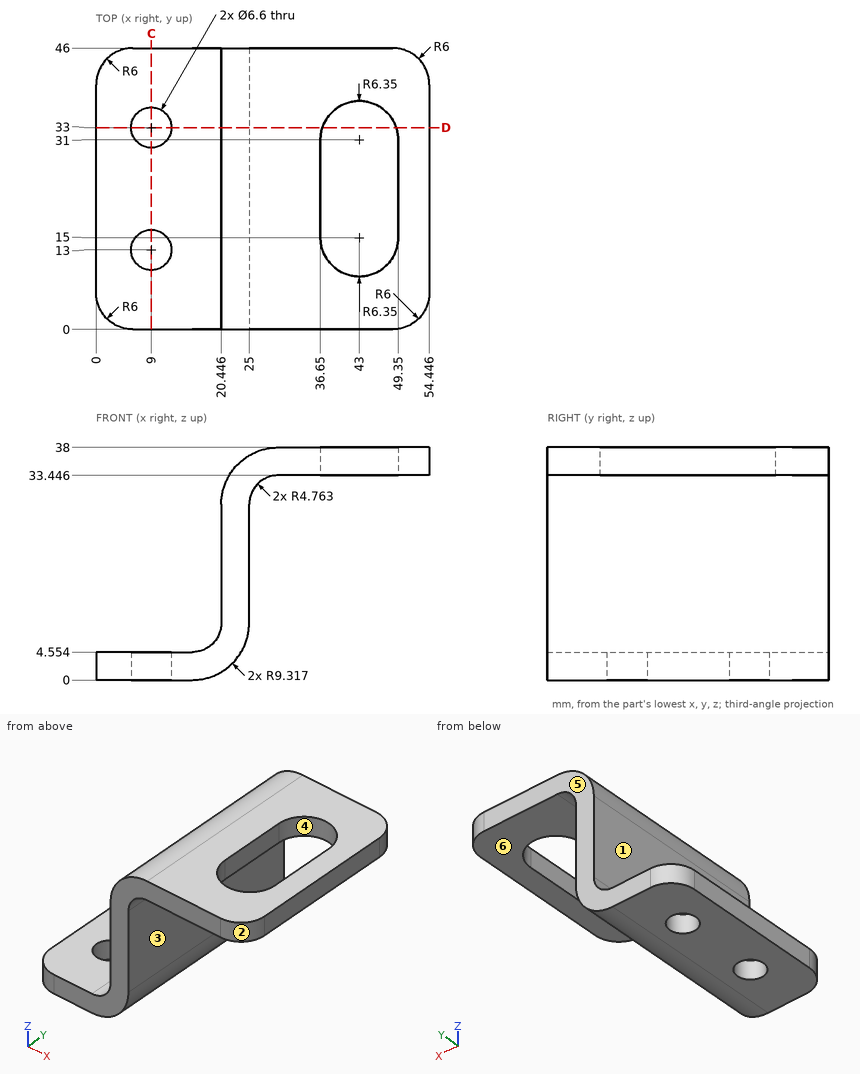
Input: dimensioned drawing with shaded views. Units: mm. Origin: part minimum x, y, z. A direction names the side the tool comes from. Give positions to 0.01 mm unless a question says otherwise; leave off trailing zeros. Write each loop counter-clockwise with the first axis right and the second up, starting at its lowest first coordinate (ties: lowest second). Pieces come first, ordered by that corner, then holes.
1. Reachability of the marked faces 1, 2 and 3 from +Z, -Z, +X, -X, +Y, -Y: full face, straight path, thin tool, end or side. Return the list, or none.
2. Section query C-C, the plane x = 9. Return loops of the section in (y, z) (1 decimal).
3. Line query: probe 1 along Y at (x, z) = (9, 2.4); probe 2 along X at (y, z) = (20, 11) (1 decimal); probe 3 along Z at (x, y) = (48, 35.5) (1 decimal). Output: solid intervals per line, ascending.
4. Section query D-D, the plane y = 33. Return loops of the section in (x, z) (1 decimal).
5. Draft query along Y for the marked faces 4, 5 and 6. Return one class per face: released by +Y, released by -Y, zero draft, split by the parting line, or undercut.
6. Pin query (flat end, axial travel): P1, Ø1.5, axis at x = 24.5, y = 23.5, coming from the +Z side (1 decimal); P2, Ø3, axis at y = 13.5, z = 31, coming from the -X side; P3, Ø3.5, axis at y = 21, z = 35, coming from the -X side. Return the tip coordinate at first contact, or that it passes through.
Computed:
1. face 1: +Z, -X, +Y, -Y
1. face 2: +Z, -Z, +X, -Y
1. face 3: -Z, +X, +Y, -Y
2. outline: (0, 0) - (9.7, 0) - (9.7, 4.6) - (0, 4.6) - close; (16.3, 0) - (29.7, 0) - (29.7, 4.6) - (16.3, 4.6) - close; (36.3, 0) - (46, 0) - (46, 4.6) - (36.3, 4.6) - close
3. probe 1: y = 0 to 9.7, 16.3 to 29.7, 36.3 to 46
3. probe 2: x = 20.4 to 25
3. probe 3: z = 33.4 to 38
4. outline: (0, 0) - (5.7, 0) - (5.7, 4.6) - (0, 4.6) - close; (12.3, 0) - (15.7, 0) arc R9.3 ccw to (25, 9.3) - (25, 28.7) arc R4.8 cw to (29.8, 33.4) - (37, 33.4) - (37, 38) - (29.8, 38) arc R9.3 ccw to (20.4, 28.7) - (20.4, 9.3) arc R4.8 cw to (15.7, 4.6) - (12.3, 4.6) - close; (49, 33.4) - (54.4, 33.4) - (54.4, 38) - (49, 38) - close
5. face 4: undercut
5. face 5: released by +Y
5. face 6: zero draft
6. P1: stops at z = 36.8
6. P2: stops at x = 20.48
6. P3: stops at x = 21.64
